Could you check a few things on this model? Use its own coordinates, in mm. A direction names the side the tool comes from. Give positions to 0.01 mm unless a question says otherwise; leave off trailing zeros. Loops run counter-clockwise (first coordinate to the right, second up) from the corner with the lowest first, then second, coordinate; pieces in that order, holes last. Notation, with made-up numbers: (13, 12.25) -> (30, 12.25) arc R17 cw to (30, 44.25) -> close; hole circle Ø10 at (-14.5, 89.5). An arc over 180 degrees is marked (long way). Write each question's results on one line, items separated by ' | '. Start each with the question number.
Q1. Will these pins go through, and if not, where does the flat tip stop? P1, Ø6.5, axis at y = 16.5, z = 10, coming from the +X side; P2, Ø5, axis at y = 19.5, z = 11, coming from the -X side; P3, Ø10, axis at x = 0, y = 11, coming from the -Z side; P4, Ø4, axis at x = -12.5, y = 18, coming from the +Z side.
Q2. Which directions (+Z, -Z, +X, -X, +Y, -Y) give clear straight access to the entire face, cutting with the end or side of a thin tool? Please do faces 5 (the face through (0, 13, 8)), 6 (the face through (0, 5, 12)), 7 (the face through (-10, 15.7, 12.1)), 8 (the face through (13, 10, 8)).
Q3. If we section it at C-C, the plane y = 3.5: List the corners of the cut face in (x, z) for me.
Q4. If we section it at B-B, the plane x = 0: List the corners of the cut face in (y, z) for me.
Q5. If I drill on line 1 along Y through (x, z) = (-8, 12); line 2 along Y through (x, z) = (12.55, 7.5); line 3 along X through (y, z) = (2.25, 11.25), over which ranges is the centre line in solid material (lowest first)?
Q6. If we section it at D-D, the plane z = 9.5: List the corners of the cut face in (x, y) for me, plus the area to 3 significant figures.
Q7. If we section it at A-A, the plane z = 2.25: List the corners of the cut face in (x, y) for me.
Q8. We'd pull the mould along X, two halves only. Please class faces 1 (the face through (15.5, 5, 8)), 2 (the face through (-13, 10, 8)), 3 (the face through (13.84, 2.96, 7.89)), 4 (the face through (-10.5, 4, 6)): released by +X, released by -X, zero draft, split by the parting line, or undercut.
from build123d import *

# Parameters (mm, degrees)
ESQUISSE1_R             = 1.4
BOSS_EXTRU_1_DEPTH      = 16
ESQUISSE2_W             = 20
ESQUISSE2_H             = 16
BOSS_EXTRU_2_DEPTH      = 15
ESQUISSE3_R             = 4
ENL_V_MAT_EXTRU_1_DEPTH = 15
ESQUISSE4_W             = 21
ESQUISSE4_H             = 8
ENL_V_MAT_EXTRU_2_DEPTH = 21
ESQUISSE5_R             = 1.4
ENL_V_MAT_EXTRU_3_DEPTH = 21


with BuildPart() as part:
    # Esquisse1 → Boss.-Extru.1 (new body)
    with BuildSketch(Plane.XY):
        Polygon((15.5, 10), (-15.5, 10), (-15.5, 0), (-10.5, 0), (-10.5, 5), (10.5, 5), (10.5, 0), (15.5, 0), align=None)
        with Locations((12.55, 3.5)):
            Circle(ESQUISSE1_R, mode=Mode.SUBTRACT)
        with Locations((-12.55, 3.5)):
            Circle(ESQUISSE1_R, mode=Mode.SUBTRACT)
    extrude(amount=BOSS_EXTRU_1_DEPTH)

    # Esquisse2 → Boss.-Extru.2 (add)
    with BuildSketch(Plane(origin=(0, 10, 0), x_dir=(1, 0, 0), z_dir=(0, 1, 0))):
        with Locations((0, -8)):
            Rectangle(ESQUISSE2_W, ESQUISSE2_H)
    extrude(amount=BOSS_EXTRU_2_DEPTH)

    # Esquisse3 → Enlèv. mat.-Extru.1 (cut)
    with BuildSketch(Plane.XY.offset(16)):
        with Locations((0, 17.5)):
            Circle(ESQUISSE3_R)
    extrude(amount=-ENL_V_MAT_EXTRU_1_DEPTH, mode=Mode.SUBTRACT)

    # Esquisse4 → Enlèv. mat.-Extru.2 (cut)
    with BuildSketch(Plane.XZ.offset(-5)):
        with Locations((0, 4)):
            Rectangle(ESQUISSE4_W, ESQUISSE4_H)
    extrude(amount=-ENL_V_MAT_EXTRU_2_DEPTH, mode=Mode.SUBTRACT)

    # Esquisse5 → Enlèv. mat.-Extru.3 (cut)
    with BuildSketch(Plane.ZY.offset(10)):
        with Locations((12, 17.5)):
            Circle(ESQUISSE5_R)
    extrude(amount=-ENL_V_MAT_EXTRU_3_DEPTH, mode=Mode.SUBTRACT)


solid = part.part
Final values:
1) P1: stops at x = 10 | P2: stops at x = -10 | P3: stops at z = 8 | P4: passes through
2) face 5: -Z, +Y, -Y | face 6: +Z, -Z, -Y | face 7: +Z, -Z, -X, +Y | face 8: +Z, -Z, +X, +Y
3) outline: (-15.5, 0) -> (-13.95, 0) -> (-13.95, 16) -> (-15.5, 16) -> close; (-11.15, 0) -> (-10.5, 0) -> (-10.5, 16) -> (-11.15, 16) -> close; (10.5, 0) -> (11.15, 0) -> (11.15, 16) -> (10.5, 16) -> close; (13.95, 0) -> (15.5, 0) -> (15.5, 16) -> (13.95, 16) -> close
4) outline: (5, 8) -> (13.5, 8) -> (13.5, 16) -> (5, 16) -> close; (21.5, 8) -> (25, 8) -> (25, 16) -> (21.5, 16) -> close
5) line 1: y = 5 to 16.1, 18.9 to 25 | line 2: y = 0 to 2.1, 4.9 to 10 | line 3: x = -15.5 to -13.18, -11.92 to -10.5, 10.5 to 11.92, 13.18 to 15.5
6) outline: (-15.5, 0) -> (-10.5, 0) -> (-10.5, 5) -> (10.5, 5) -> (10.5, 0) -> (15.5, 0) -> (15.5, 10) -> (10, 10) -> (10, 25) -> (-10, 25) -> (-10, 10) -> (-15.5, 10) -> close; hole circle Ø2.8 at (-12.55, 3.5); hole circle Ø8 at (0, 17.5); hole circle Ø2.8 at (12.55, 3.5) | area: 442 mm²
7) outline: (-15.5, 0) -> (-10.5, 0) -> (-10.5, 10) -> (-15.5, 10) -> close; (10.5, 0) -> (15.5, 0) -> (15.5, 10) -> (10.5, 10) -> close; hole circle Ø2.8 at (-12.55, 3.5); hole circle Ø2.8 at (12.55, 3.5)
8) face 1: released by +X | face 2: zero draft | face 3: undercut | face 4: undercut
